from build123d import *

# Parameters (mm, degrees)
SKETCH_R              = 17.5
PAD_DEPTH             = 3.4
FILLET_R              = 1
SKETCH001_R           = 15.5
SKETCH001_R_2         = 13.5
PAD001_DEPTH          = 22
CHAMFER_SIZE2         = 1
CHAMFER_SIZE          = 3
POCKET_DEPTH          = 22
POLARPATTERN_COUNT    = 4
PAD002_DEPTH          = 10
POLARPATTERN001_COUNT = 4
SKETCH006_R           = 12.5
SKETCH005_R           = 9.5
SKETCH007_R           = 6
POCKET001_DEPTH       = 36.401
FILLET001_R           = 3
CHAMFER002_SIZE2      = 0.4
CHAMFER002_SIZE       = 1
PAD003_DEPTH          = 12
POLARPATTERN002_COUNT = 4


with BuildPart() as part:
    # Sketch (on XY_Plane of Origin) → Pad (new body)
    with BuildSketch(Plane.XY):
        Circle(SKETCH_R)
    extrude(amount=PAD_DEPTH)

    # Fillet
    fillet_edges = [part.edges().sort_by_distance(p)[0] for p in [
        (-17.5, 0, 3.4),
    ]]
    fillet(fillet_edges, radius=FILLET_R)

    # Sketch001 (on Face3 of Fillet) → Pad001 (join)
    with BuildSketch(Plane(origin=(0, 0, 0), x_dir=(1, 0, 0), z_dir=(0, 0, -1))):
        Circle(SKETCH001_R)
        Circle(SKETCH001_R_2, mode=Mode.SUBTRACT)
    extrude(amount=PAD001_DEPTH)

    # Chamfer
    chamfer_edges = [part.edges().sort_by_distance(p)[0] for p in [
        (-15.5, 0, -22),
    ]]
    chamfer_side = part.faces().sort_by_distance((-15.5, 0, -11))[0]
    chamfer(chamfer_edges, length=CHAMFER_SIZE, length2=CHAMFER_SIZE2, reference=chamfer_side)

    # Sketch003 (on Face3 of Chamfer) → Pocket (cut)
    with BuildSketch(Plane(origin=(0, 0, 0), x_dir=(1, 0, 0), z_dir=(0, 0, -1))):
        with BuildLine():
            ThreePointArc((2.929699, 16.745652), (-0.022663, 16.999985), (-2.974337, 16.737781))
            Line((-2.974337, 16.737781), (-2.170603, 12.310097))
            ThreePointArc((2.170603, 12.310097), (0, 12.5), (-2.170603, 12.310097))
            Line((2.929699, 16.745652), (2.170603, 12.310097))
        make_face()
    pocket = extrude(amount=POCKET_DEPTH, mode=Mode.SUBTRACT)

    # PolarPattern: Pocket ×4 about axis
    polarpattern_axis = Axis((0, 0, 0), (0, 0, -1))
    for i in range(1, POLARPATTERN_COUNT):
        add(pocket.rotate(polarpattern_axis, i * 360 / POLARPATTERN_COUNT), mode=Mode.SUBTRACT)

    # Sketch004 → Pad002 (join)
    with BuildSketch(Plane(origin=(0, 0, -9), x_dir=(0.707107, 0.707107, 0), z_dir=(0, 0, 1))):
        with BuildLine():
            ThreePointArc((0.31147, 15.49687), (-0.094297, 15.499713), (-0.5, 15.491933))
            ThreePointArc((0.31147, 15.49687), (-0.095665, 15.724518), (-0.5, 15.491933))
        make_face()
    pad002 = extrude(amount=PAD002_DEPTH)

    # PolarPattern001: Pad002 ×4 about axis
    polarpattern001_axis = Axis((0, 0, -9), (0, 0, 1))
    for i in range(1, POLARPATTERN001_COUNT):
        add(pad002.rotate(polarpattern001_axis, i * 360 / POLARPATTERN001_COUNT))

    # Sketch006 (on Face3 of PolarPattern001) → AdditiveLoft section 0
    with BuildSketch(Plane(origin=(0, 0, 0), x_dir=(1, 0, 0), z_dir=(0, 0, -1))):
        Circle(SKETCH006_R)
    # Sketch005 (on Face3 of PolarPattern001) → AdditiveLoft section 1
    with BuildSketch(Plane(origin=(0, 0, -33), x_dir=(1, 0, 0), z_dir=(0, 0, -1))):
        Circle(SKETCH005_R)
    loft()

    # Sketch007 (on Face32 of AdditiveLoft) → Pocket001 (cut, through all)
    with BuildSketch(Plane(origin=(0, 0, -33), x_dir=(1, 0, 0), z_dir=(0, 0, -1))):
        Circle(SKETCH007_R)
    extrude(amount=-POCKET001_DEPTH, mode=Mode.SUBTRACT)

    # Fillet001
    fillet001_edges = [part.edges().sort_by_distance(p)[0] for p in [
        (-9.5, 0, -33),
    ]]
    fillet(fillet001_edges, radius=FILLET001_R)

    # Chamfer002
    chamfer002_edges = [part.edges().sort_by_distance(p)[0] for p in [
        (-6, 0, 3.4),
    ]]
    chamfer002_side = part.faces().sort_by_distance((-6, 0, -14.8))[0]
    chamfer(chamfer002_edges, length=CHAMFER002_SIZE, length2=CHAMFER002_SIZE2, reference=chamfer002_side)

    # Sketch008 (on Face9 of Chamfer002) → Pad003 (join)
    with BuildSketch(Plane(origin=(0, 0, 0), x_dir=(0.087156, -0.996195, 0), z_dir=(0, 0, -1))):
        with BuildLine():
            ThreePointArc((-9.880104, 9.918848), (-10.706992, 9.019996), (-11.452393, 8.052496))
            Line((-11.452393, 8.052496), (-7.356621, 5.184605))
            ThreePointArc((-6.344559, 6.383304), (-6.876758, 5.806048), (-7.356621, 5.184605))
            Line((-6.344559, 6.383304), (-9.880104, 9.918848))
        make_face()
    pad003 = extrude(amount=PAD003_DEPTH)

    # PolarPattern002: Pad003 ×4 about axis
    polarpattern002_axis = Axis((0, 0, 0), (0, 0, -1))
    for i in range(1, POLARPATTERN002_COUNT):
        add(pad003.rotate(polarpattern002_axis, i * 360 / POLARPATTERN002_COUNT))


solid = part.part
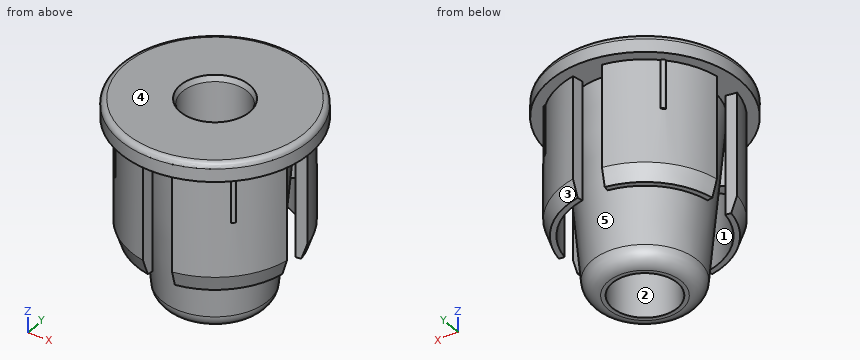
Could you check a few things on this model? Use its own coordinates, in mm. Face numbers are marked on the shaded views. A direction names the side the tool comes from. Coordinates: 2 decimals unless noted, no trailing zeros. Order: outer loops, then holes, each group sorted by start corner. A loop starts at its lowest first (then second) coordinate and runs counter-clockwise, first axis right, second up. Notation, with made-up numbers: (14.25, 60) -> (26.25, 60) arc R22 cw to (26.25, 77) -> close; hole circle Ø2 at (28, 76.25). An arc over 180 degrees is marked (long way). One line per item, written item: value. Start each with the question number.
1) Imagine slicing it at A-A on x = 0. List the corners of the cut face in (y, z) for me, plus the area to 3 significant figures.
2) Imagine slicing it at B-B on z = -15. List the corners of the cut face in (x, y) for me, plus the area to 3 significant figures.
3) Which directions (+Z, -Z, +X, -X, +Y, -Y) give clear straight access to the entire face, cutting with the end or side of a thin tool? Please do the marked faces 1 and 2.
4) We'd pull the mould along X, two halves only. Please class the marked faces 3, 4 and 5: +X half, -X half, draft (parallel to the pull), parting line (faces both ways), or undercut.
5) I'm going to push flat-ended pins straight in: pin 1 (4 mm diameter, centred on y = -12.5, z = -27, fed in from +X); pin 2 (4 mm diameter, centred on x = -8, y = 11, fed in from -Z); pin 3 (3.5 mm diameter, centred on x = -9.5, y = 6, fed in from -Z); pin 4 (0.9 mm diameter, centred on x = 8, y = 9.5, fed in from -Z). Where does each tip first touch, or does it pass through?
Answer list:
1. outline: (-17.5, 0) -> (-12.5, 0) -> (-9.75, -30.27) arc R3 ccw to (-6.76, -33) -> (-6, -33) -> (-6, 2.4) -> (-6.4, 3.4) -> (-16.5, 3.4) arc R1 ccw to (-17.5, 2.4) -> close; (6, -33) -> (6.76, -33) arc R3 ccw to (9.75, -30.27) -> (12.5, 0) -> (17.5, 0) -> (17.5, 2.4) arc R1 ccw to (16.5, 3.4) -> (6.4, 3.4) -> (6, 2.4) -> close
1. area: 404 mm2
2. outline: (-15.27, -2.68) arc R15.5 ccw to (-2.71, -15.26) -> (-2.35, -13.29) arc R13.5 cw to (-13.3, -2.34) -> close; (-15.26, 2.71) -> (-13.29, 2.35) arc R13.5 cw to (-2.34, 13.3) -> (-2.68, 15.27) arc R15.5 ccw to start; circle Ø22.27 at (0, 0); (2.34, -13.3) -> (2.68, -15.27) arc R15.5 ccw to (15.26, -2.71) -> (13.29, -2.35) arc R13.5 cw to start; (2.35, 13.29) arc R13.5 cw to (13.3, 2.34) -> (15.27, 2.68) arc R15.5 ccw to (2.71, 15.26) -> close; hole circle Ø12 at (0, 0)
2. area: 418 mm2
3. face 1: -Z
3. face 2: +Z, -Z
4. face 3: +X half
4. face 4: draft
4. face 5: undercut
5. pin 1: passes through
5. pin 2: stops at z = -22
5. pin 3: stops at z = -31.25
5. pin 4: stops at z = -12
